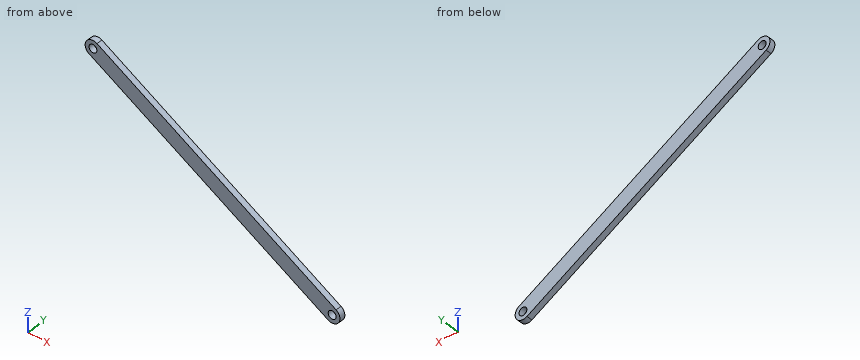
Autodesk Inventor part; units mm, degrees
ref_plane "YZ Plane" through (0, 0, 0) normal (1, 0, 0) x (0, 1, 0)
ref_plane "XZ Plane" through (0, 0, 0) normal (0, 1, 0) x (-1, 0, 0)
ref_plane "XY Plane" through (0, 0, 0) normal (0, 0, 1) x (1, 0, 0)
ref_plane "Work Plane1" through (-47.4023, 137.8054, 11.1867) normal (0, 1, 0) x (-1, 0, 0)
sketch "Sketch1" plane through (-47.4023, 137.8054, 11.1867) normal (0, 1, 0) x (-1, 0, 0)
  line L0 (13.9385, 9.5711) -> (4.3301, -7.0711)
  line L1 (-13.9385, 9.5711) -> (13.9385, 9.5711)
  line L2 (-4.3301, -7.0711) -> (-13.9385, 9.5711)
  arc A0 (-4.3301, -7.0711) -> (4.3301, -7.0711) centre (0, -4.5711) ccw
  circle A1 centre (0, -4.5711) radius 2
  line L3 (-115.8579, -75.4289) -> (-115.8579, -90.4289)
  arc A2 (-115.8579, -75.4289) -> (-120.8579, -70.4289) centre (-120.8579, -75.4289) ccw
  line L4 (-135.8579, -70.4289) -> (-120.8579, -70.4289)
  line L5 (-135.8579, -90.4289) -> (-135.8579, -70.4289)
  line L6 (-115.8579, -90.4289) -> (-135.8579, -90.4289)
  circle A3 centre (-121.7157, -76.2868) radius 2
  line L7 (-121.7157, -76.2868) -> (0, -4.5711) construction
  line L8 (-119.6852, -79.7331) -> (2.0306, -8.0173)
  line L9 (-2.0306, -1.1248) -> (-123.7463, -72.8405)
  arc A4 (-123.7463, -72.8405) -> (-119.6852, -79.7331) centre (-121.7157, -76.2868) ccw
  arc A5 (2.0306, -8.0173) -> (-2.0306, -1.1248) centre (0, -4.5711) ccw
  point P0 (-47.4023, -11.1867)
  point P1 (-60.8579, -40.4289)
  dimension "d0" = 8
extrude "Extrusion1" add sketch "Sketch1" along normal blind 3 contours L8 L3 A2 L9 L2 A0 | A0 L2 L9 A5 L8 | L8 A4 L9 A2 L3
properties part number "truss final piece"
CAD build for the part. Positions are in the model's coordinates, mm. Round coordinates to 2 decimals unless told otherwise and drop trailing zeros. Order: outer loops, then holes, each group sorted by start corner. A loop starts at its lowest first (then second) coordinate and runs counter-clockwise, first axis right, second up. Notation, with made-up numbers: (-20, 58.25) -> (17, 58.25) arc R32 cw to (17, 84.25) -> close; hole circle Ø8 at (13.25, -7.75). An arc over 180 degrees is marked (long way). Write item = value, one per line. Start each with the question number.
(1) Probe line 1 (X direction, y = 140.35, z = 5); line 2 (Z direction, x = -0.5, y = 138.7); line 3 (Z direction, x = 33.5, y = 139). List the from-to ranges inside material, lowest first. Write a range as [from, to].
(2) Cut at A-A, the plane y = 138.8. List the corners of the cut face in (x, z).
(3) Cut at C-C, the plane z = -21. List the corners of the cut face in (x, y), then the cut area to 3 significant figures.
(4) Pin check, flat tips, straight feed: P1, Ø1, axis at x = 30.5, y = 138.5, coming from the -Z side; P2, Ø5, axis at x = 74.31, z = -65.1, coming from the -Y side; P3, Ø1.5, axis at x = 3, y = 139, coming from the -Z side; P4, Ø1, axis at y = 140.5, z = -41.5, coming from the -X side. Stop position of each tip, or through.
(5) Cut at B-B, the plane x = 49.5. List the corners of the cut face in (y, z).
Model answer:
q1.line_1 = [-51.06, -48.58], [-46.22, -36.78]
q1.line_2 = [-25.66, -16.38]
q1.line_3 = [-45.7, -36.41]
q2.outline = (-49.43, 3.17) -> (72.28, -68.55) arc R4 ccw to (76.34, -61.65) -> (-45.37, 10.06) arc R4 ccw to start; hole circle Ø4 at (-47.4, 6.62); hole circle Ø4 at (74.31, -65.1)
q3.outline = (-8.41, 137.81) -> (7.35, 137.81) -> (7.35, 140.81) -> (-8.41, 140.81) -> close
q3.area = 47.3 mm2
q4.P1 = -44.22
q4.P2 = 137.81
q4.P3 = -28.17
q4.P4 = 25.53
q5.outline = (137.81, -55.12) -> (140.81, -55.12) -> (140.81, -45.84) -> (137.81, -45.84) -> close
